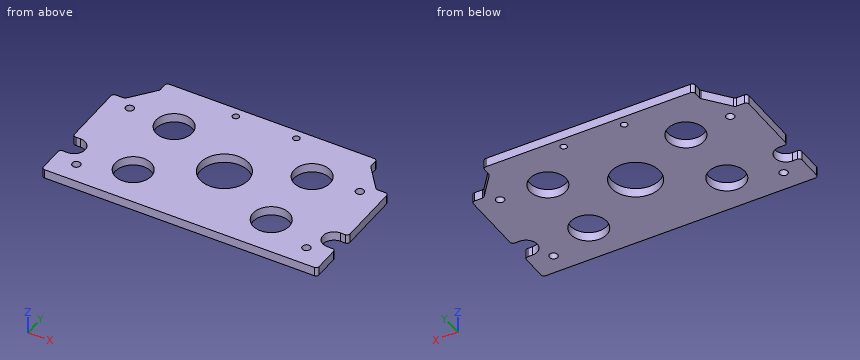
from build123d import *

# Parameters (mm, degrees)
BOSS_EXTRUDE1_DEPTH         = 4.7625
F_6_CLEARANCE_HOLE1_D       = 4.3053
F_3_4_0_75_DIAMETER_HOLE1_D = 19.05
F_1_1_DIAMETER_HOLE1_D      = 25.4
F_4_CLEARANCE_HOLE1_D       = 3.4544


with BuildPart() as part:
    # Sketch1 → Boss-Extrude1 (new body)
    with BuildSketch(Plane.XY):
        with BuildLine():
            Line((0.762, 54.483), (0.762, 41.5925))
            ThreePointArc((0.762, 41.5925), (1.226967985, 40.469967985), (2.3495, 40.005))
            Line((2.3495, 40.005), (143.7005, 40.005))
            ThreePointArc((143.7005, 40.005), (144.823032015, 40.469967985), (145.288, 41.5925))
            Line((145.288, 41.5925), (145.288, 54.483))
            ThreePointArc((145.288, 54.483), (144.823032015, 55.605532015), (143.7005, 56.0705))
            Line((143.7005, 56.0705), (141.1605, 56.0705))
            ThreePointArc((141.1605, 56.0705), (135.3185, 61.9125), (141.1605, 67.7545))
            Line((141.1605, 67.7545), (143.7005, 67.7545))
            ThreePointArc((143.7005, 67.7545), (144.823032015, 68.219467985), (145.288, 69.342))
            Line((145.288, 69.342), (145.288, 101.9175))
            ThreePointArc((145.288, 101.9175), (144.823032015, 103.040032015), (143.7005, 103.505))
            Line((143.7005, 103.505), (139.696431174, 103.505))
            ThreePointArc((139.696431174, 103.505), (139.012088949, 103.660078285), (138.46144955, 104.095014842))
            Line((138.46144955, 104.095014842), (128.622518376, 116.276548677))
            ThreePointArc((128.622518376, 116.276548677), (128.360721864, 116.745061754), (128.27, 117.274033834))
            Line((128.27, 117.274033834), (128.27, 120.9675))
            ThreePointArc((128.27, 120.9675), (127.805032015, 122.090032015), (126.6825, 122.555))
            Line((126.6825, 122.555), (19.3675, 122.555))
            ThreePointArc((19.3675, 122.555), (18.244967985, 122.090032015), (17.78, 120.9675))
            Line((17.78, 120.9675), (17.78, 117.274033834))
            ThreePointArc((17.78, 117.274033834), (17.689278136, 116.745061754), (17.427481624, 116.276548677))
            Line((17.427481624, 116.276548677), (7.58855045, 104.095014842))
            ThreePointArc((7.58855045, 104.095014842), (7.037911051, 103.660078285), (6.353568826, 103.505))
            Line((6.353568826, 103.505), (2.3495, 103.505))
            ThreePointArc((2.3495, 103.505), (1.226967985, 103.040032015), (0.762, 101.9175))
            Line((0.762, 101.9175), (0.762, 69.342))
            ThreePointArc((0.762, 69.342), (1.226967985, 68.219467985), (2.3495, 67.7545))
            Line((2.3495, 67.7545), (4.8895, 67.7545))
            ThreePointArc((4.8895, 67.7545), (10.7315, 61.9125), (4.8895, 56.0705))
            Line((4.8895, 56.0705), (2.3495, 56.0705))
            ThreePointArc((2.3495, 56.0705), (1.226967985, 55.605532015), (0.762, 54.483))
        make_face()
    extrude(amount=BOSS_EXTRUDE1_DEPTH)

    # #6 Clearance Hole1 (through all)
    with Locations(Plane.XY.offset(4.7625)):
        with Locations((12.7, 98.425), (133.35, 98.425), (133.35, 50.673), (12.7, 50.673)):
            Hole(F_6_CLEARANCE_HOLE1_D / 2)

    # 3/4 (0.75) Diameter Hole1 (through all)
    with Locations(Plane.XY.offset(4.7625)):
        with Locations((36.83, 96.901), (109.22, 96.901), (109.22, 60.325), (36.83, 60.325)):
            Hole(F_3_4_0_75_DIAMETER_HOLE1_D / 2)

    # 1 (1) Diameter Hole1 (through all)
    with Locations(Plane.XY.offset(4.7625)):
        with Locations((73.025, 80.137)):
            Hole(F_1_1_DIAMETER_HOLE1_D / 2)

    # #4 Clearance Hole1 (through all)
    with Locations(Plane.XY.offset(4.7625)):
        with Locations((57.15, 117.475), (88.9, 117.475)):
            Hole(F_4_CLEARANCE_HOLE1_D / 2)


solid = part.part
Model file for the job. Use its own axes, mm. Coordinates: 2 decimals unless noted, no trailing zeros. Order: outer loops, then holes, each group sorted by start corner. A loop starts at its lowest first (then second) coordinate and runs counter-clockwise, first axis right, second up. Notation, with made-up numbers: (-39, 86.25) -> (-12, 86.25) arc R20 cw to (-12, 124.25) -> close; hole circle Ø6 at (57.5, 33.25). An arc over 180 degrees is marked (long way). Return JSON: item names as keys, results as strings. Group by question number.
Item 1: Saw through at C-C on y = 57.5. Write the cut outline in (x, z), then the cut area to 3 significant figures.
Item 2: Flat gauge pins, fed straight in: P1, Ø2, axis at x = 141.5, z = 3, coming from the +Y side (3 decimals); P2, Ø2, axis at y = 106.5, z = 1, coming from the +X side; P3, Ø1.1, axis at y = 118.5, z = 1, coming from the -X side. Where does each tip first touch, or does it go through?
Item 3: Saw through at A-A on x = 109.22. State how many separate pieces and enclosed holes the cut face has, then the cut area to 3 significant figures.
Item 4: Wall check: line 1 along Y through (x, z) = (37, 0.4) (3 decimals); line 2 along X through (y, z) = (55, 4); line 3 along Y through (x, z) = (133.35, 2.95) (3 decimals). Give the ranges that are in metal, low to high. Write a range as [from, to].
Item 5: Saw through at B-B on x = 57.15. Write the cut outline in (y, z) (1 decimal), then the cut area to 3 significant figures.
Values found:
{
 "1": {"outline": "(8.72, 0) -> (27.73, 0) -> (27.73, 4.76) -> (8.72, 4.76) -> close; (45.93, 0) -> (100.12, 0) -> (100.12, 4.76) -> (45.93, 4.76) -> close; (118.32, 0) -> (137.33, 0) -> (137.33, 4.76) -> (118.32, 4.76) -> close", "area": "439 mm2"},
 "2": {"P1": "stops at y = 103.505", "P2": "stops at x = 137.33", "P3": "stops at x = 17.78"},
 "3": {"separate pieces": "3", "enclosed holes": "0", "area": "212 mm2"},
 "4": {"line 1": "y = [40.005, 50.802], [69.848, 87.378], [106.424, 122.555]", "line 2": "x = [0.85, 28.93], [44.73, 101.32], [117.12, 145.2]", "line 3": "y = [40.005, 48.52], [52.826, 96.272], [100.578, 110.423]"},
 "5": {"outline": "(40, 0) -> (115.7, 0) -> (115.7, 4.8) -> (40, 4.8) -> close; (119.2, 0) -> (122.6, 0) -> (122.6, 4.8) -> (119.2, 4.8) -> close", "area": "377 mm2"}
}
